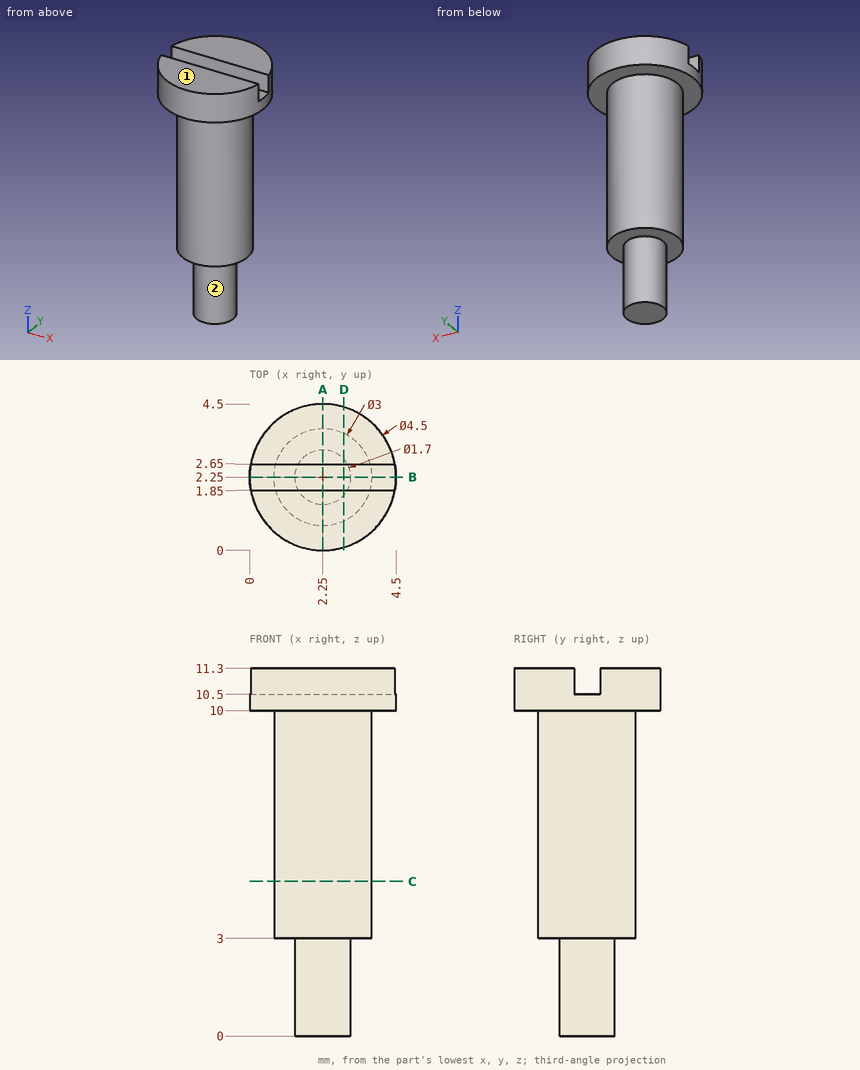
For this review, use the dimensioned drawing (mm, ordinates from the lowest corner) and the shaded views. A direction names the side the tool comes from. Round coordinates to 2 decimals unless told otherwise and drop trailing zeros. Write each loop counter-clockwise with the first axis right and the second up, starting at its lowest first coordinate (ties: lowest second). Pieces come first, ordered by that corner, then holes. Notation, with made-up numbers: (7, 29.5) - (35, 29.5) arc R5 cw to (35, 33.5) - close; hole circle Ø4 at (49, 84). An arc over 180 degrees is marked (long way). Use a Markdown table: item, result.
Q1. We need section D-D (x = 2.9). Give the boundary of the cut face in (y, z).
Derived:
| item | result |
|---|---|
| outline | (0.1, 10) - (0.9, 10) - (0.9, 3) - (1.7, 3) - (1.7, 0) - (2.8, 0) - (2.8, 3) - (3.6, 3) - (3.6, 10) - (4.4, 10) - (4.4, 11.3) - (2.65, 11.3) - (2.65, 10.5) - (1.85, 10.5) - (1.85, 11.3) - (0.1, 11.3) - close |
Q2. We need section B-B (y = 2.25). Give the boundary of the cut face in (x, z).
Derived:
| item | result |
|---|---|
| outline | (0, 10) - (0.75, 10) - (0.75, 3) - (1.4, 3) - (1.4, 0) - (3.1, 0) - (3.1, 3) - (3.75, 3) - (3.75, 10) - (4.5, 10) - (4.5, 10.5) - (0, 10.5) - close |
Q3. Machinability: for the marked faces 1 and 2, which of the approach directions +Z, -Z, +X, -X, +Y, -Y give a long, thin tool a straight path to every point of the face, cutting with its end or side? Answer none if there is none.
Derived:
| item | result |
|---|---|
| face 1 | +Z, +X, -X, +Y, -Y |
| face 2 | -Z |
Q4. We need section A-A (x = 2.25). Give the boundary of the cut face in (y, z), plus the area to 3 significant figures.
Derived:
| item | result |
|---|---|
| outline | (0, 10) - (0.75, 10) - (0.75, 3) - (1.4, 3) - (1.4, 0) - (3.1, 0) - (3.1, 3) - (3.75, 3) - (3.75, 10) - (4.5, 10) - (4.5, 11.3) - (2.65, 11.3) - (2.65, 10.5) - (1.85, 10.5) - (1.85, 11.3) - (0, 11.3) - close |
| area | 31.3 mm2 |
Q5. Wall thickness on line 1 along Z through (x, y) = (0.35, 1.7); line 2 along Z through (x, y) = (1.9, 1.15); line 3 along Y through (x, z) = (2.55, 11.25): over which ranges is each line inside the solid? List them lowest first.
Derived:
| item | result |
|---|---|
| line 1 | z = 10 to 11.3 |
| line 2 | z = 3 to 11.3 |
| line 3 | y = 0.02 to 1.85, 2.65 to 4.48 |
Q6. We need section C-C (z = 4.75). Give the boundary of the cut face in (x, y), plus the area to 3 significant figures.
Derived:
| item | result |
|---|---|
| outline | circle Ø3 at (2.25, 2.25) |
| area | 7.07 mm2 |
Q7. Clearance check with flat-ended pins moving along their axes: pin 1 (0.9 mm diameter, centred on x = 3, z = 11, fed in from +Y); pin 2 (0.9 mm diameter, centred on x = 1, z = 11, fed in from -Y). State where each tip first meets the part, or that it passes through.
Derived:
| item | result |
|---|---|
| pin 1 | stops at y = 4.48 |
| pin 2 | stops at y = 0.15 |
